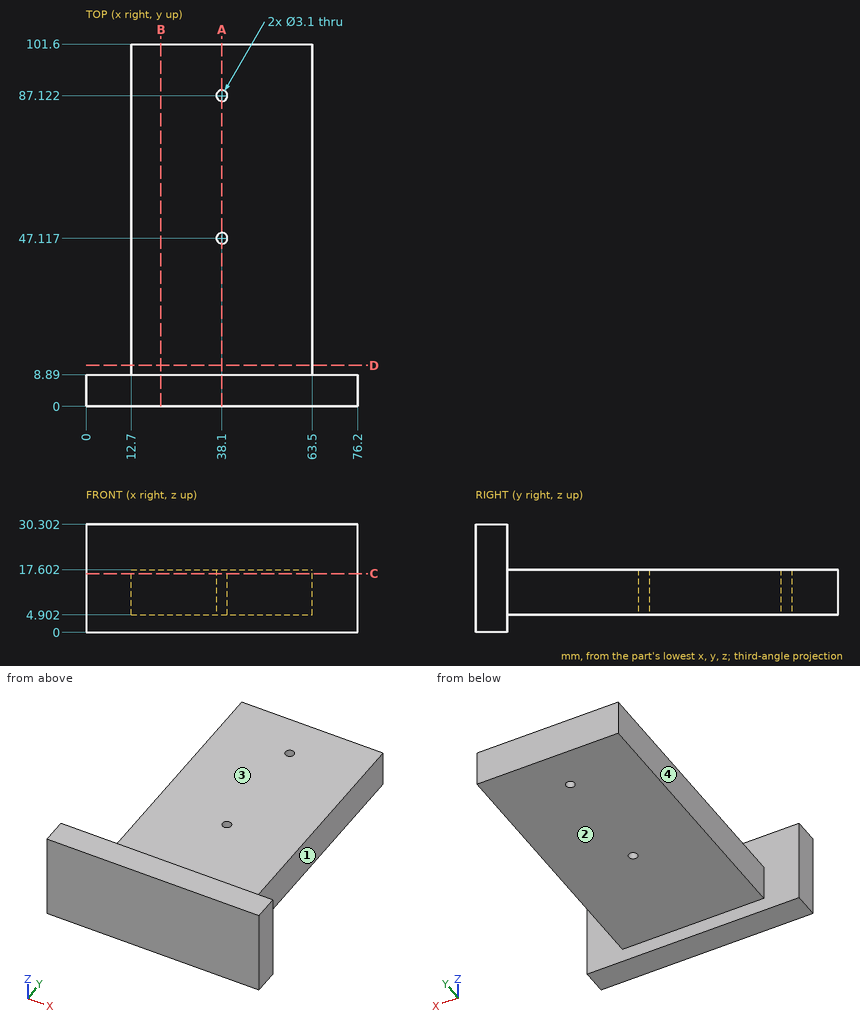
Verification items for this drawing (mm, ordinates from the low corner). A direction names the side the tool comes from. Coordinates: 2 decimals unless noted, no trailing zeros. Loops run counter-clockwise (first coordinate to the right, second up) from the corner with the lowest first, then second, coordinate; pieces in that order, holes last. Notation, with made-up numbers: (-35.75, 22) -> (8.25, 22) arc R22 cw to (8.25, 47) -> close; hole circle Ø8 at (-11.5, 60). An arc over 180 degrees is marked (long way). Answer in a Markdown table with one row per item. Add a question column.
1. Depth check by flat-ended pin: P1, Ø4, axis at x = 12, z = 11.5, coming from the +Y side; P2, Ø3.5, axis at x = 38.1, y = 47.117, coming from the +Z side; P3, Ø6.5, axis at y = 38.5, z = 13.5, coming from the +X side; P4, Ø6.5, axis at y = 45.5, z = 10, coming from the -X side. Enter the tip coordinate at first touch or a pass-through.
2. Access from +Z, -Z, +X, -X, +Y, -Y to the whole of each face (thin tool, end or side, straight path). Record for the marked faces 1, 2, 3 and 4.
3. Section check B-B, the plane x = 21. Enter the section's corners in (y, z).
4. Section check A-A, the plane x = 38.1. Enter the section's corners in (y, z).
5. Material ranges on probe 1 along Y at (x, z) = (38.1, 13.5); probe 2 along Y at (x, z) = (67.5, 11); probe 3 along X at (y, z) = (64, 13.5), recorded low to high. Write a range as [from, to].
6. Section check D-D, the plane y = 11.5. Enter the section's corners in (x, z).
7. Section check C-C, the plane z = 16.5. Enter the section's corners in (x, y), then the cut area to 3 significant figures.
Derived:
| question | item | result |
|---|---|---|
| 1 | P1 | stops at y = 101.6 |
| 1 | P2 | stops at z = 17.6 |
| 1 | P3 | stops at x = 63.5 |
| 1 | P4 | stops at x = 12.7 |
| 2 | face 1 | +Z, -Z, +X, +Y |
| 2 | face 2 | -Z, +X, -X, +Y |
| 2 | face 3 | +Z, +X, -X, +Y |
| 2 | face 4 | +Z, -Z, -X, +Y |
| 3 | outline | (0, 0) -> (8.89, 0) -> (8.89, 4.9) -> (101.6, 4.9) -> (101.6, 17.6) -> (8.89, 17.6) -> (8.89, 30.3) -> (0, 30.3) -> close |
| 4 | outline | (0, 0) -> (8.89, 0) -> (8.89, 4.9) -> (45.57, 4.9) -> (45.57, 17.6) -> (8.89, 17.6) -> (8.89, 30.3) -> (0, 30.3) -> close; (48.67, 4.9) -> (85.57, 4.9) -> (85.57, 17.6) -> (48.67, 17.6) -> close; (88.67, 4.9) -> (101.6, 4.9) -> (101.6, 17.6) -> (88.67, 17.6) -> close |
| 5 | probe 1 | y = [0, 45.57], [48.67, 85.57], [88.67, 101.6] |
| 5 | probe 2 | y = [0, 8.89] |
| 5 | probe 3 | x = [12.7, 63.5] |
| 6 | outline | (12.7, 4.9) -> (63.5, 4.9) -> (63.5, 17.6) -> (12.7, 17.6) -> close |
| 7 | outline | (0, 0) -> (76.2, 0) -> (76.2, 8.89) -> (63.5, 8.89) -> (63.5, 101.6) -> (12.7, 101.6) -> (12.7, 8.89) -> (0, 8.89) -> close; hole circle Ø3.1 at (38.1, 47.12); hole circle Ø3.1 at (38.1, 87.12) |
| 7 | area | 5,370 mm² |
